Source: CAD feature listing. Evaluate the final solid. Frame: model axes, mm. A direction names the side the tool comes from. Round coordinates to 2 decimals unless told otherwise and drop trailing zeros. Order: outer loops, then holes, each group sorted by start corner. A loop starts at its lowest first (then second) coordinate and runs counter-clockwise, first axis right, second up. Notation, with made-up numbers: (25.25, -21.5) - (55.25, -21.5) arc R17 ccw to (55.25, -17.5) - close; hole circle Ø1 at (82.25, -18.5). An arc over 180 degrees is marked (long way). Use one line per item in the form item = value. Start each with the question number.
Q1. Cut plane A-A, the plane z = 0. Return the cut outline in (x, y).
Q2. Ray query, line 1 (Y direction, x = -1.25, z = 6.5); line 2 (X direction, y = 22, z = -0.5); line 3 (Z direction, x = -0.25, y = -14). Return the intervals inside material, ascending. Write a range as [from, to].
Q3. Pin query (flat end, axial travel): pin 1 Ø4 at (y, z) = (-22.5, 7.5) entering from +X; pin 2 Ø4 at (x, y) = (-3, 24) entering from +Z; pin 3 Ø10 at (y, z) = (-26.5, 6) entering from +X. Return the tip coordinate at first contact, or that it passes through.
Q4. Cut plane B-B, the plane x = 0. Return the cut outline in (y, z), and give its area (3 significant figures).
Q5. Set-up query: faces 1 (the cylindrical face through (10, 0, 0)), 2 (the flat face through (4, 30, 4)), 3 (the flat face through (-4, -30, 4)). Return all of +Z, -Z, +X, -X, +Y, -Y with unobstructed straight access to the full face (end or side cutting, diameter ignored); none if empty.
Q6. Cut plane C-C, the plane y = 11.5. Return the cut outline in (x, z).
from build123d import *

# Parameters (mm, degrees)
CHAMFER_1_SIZE = 1
CHAMFER_2_SIZE = 0.2


with BuildPart() as part:
    # 草图1 → 旋转1 (revolve)
    with BuildSketch(Plane.XY, mode=Mode.PRIVATE) as revolve_1_sk:
        Polygon((0, 40), (5, 40), (5, 30), (10, 30), (10, -30), (5, -30), (5, -40), (0, -40), align=None)
    revolve(revolve_1_sk.sketch.rotate(Axis((0, 40, 0), (0, -1, 0)), 180), axis=Axis((0, 40, 0), (0, -1, 0)))

    # 倒角1
    chamfer_1_edges = [part.edges().sort_by_distance(p)[0] for p in [
        (5, -40, 0),
        (10, -30, 0),
        (10, 30, 0),
        (5, 40, 0),
    ]]
    chamfer(chamfer_1_edges, length=CHAMFER_1_SIZE)

    # 倒角2
    chamfer_2_edges = [part.edges().sort_by_distance(p)[0] for p in [
        (5, -30, 0),
        (5, 30, 0),
    ]]
    chamfer(chamfer_2_edges, length=CHAMFER_2_SIZE)


solid = part.part
Completed:
q1.outline = (-10, -29) - (-9, -30) - (-5.2, -30) - (-5, -30.2) - (-5, -39) - (-4, -40) - (4, -40) - (5, -39) - (5, -30.2) - (5.2, -30) - (9, -30) - (10, -29) - (10, 29) - (9, 30) - (5.2, 30) - (5, 30.2) - (5, 39) - (4, 40) - (-4, 40) - (-5, 39) - (-5, 30.2) - (-5.2, 30) - (-9, 30) - (-10, 29) - close
q2.line_1 = [-30, 30]
q2.line_2 = [-9.99, 9.99]
q2.line_3 = [-10, 10]
q3.pin_1 = 8.35
q3.pin_2 = 9.95
q3.pin_3 = 9.95
q4.outline = (-40, -4) - (-39, -5) - (-30.2, -5) - (-30, -5.2) - (-30, -9) - (-29, -10) - (29, -10) - (30, -9) - (30, -5.2) - (30.2, -5) - (39, -5) - (40, -4) - (40, 4) - (39, 5) - (30.2, 5) - (30, 5.2) - (30, 9) - (29, 10) - (-29, 10) - (-30, 9) - (-30, 5.2) - (-30.2, 5) - (-39, 5) - (-40, 4) - close
q4.area = 1,400 mm2
q5.face_1 = +Y, -Y
q5.face_2 = +Y
q5.face_3 = -Y
q6.outline = circle Ø20 at (0, 0)
